Here's the drawing with two shaded views (mm, measured from the low corner). I have some questions. Give positions to 0.01 mm unless a question says otherwise; leave off trailing zeros. Write each loop counter-clockwise with the first axis right and the second up, starting at its lowest first coordinate (ties: lowest second). Pieces come first, ordered by that corner, then holes. Notation, with made-up numbers: (-8.5, 47.5) -> (12.5, 47.5) arc R16 ccw to (12.5, 76.5) -> close; hole circle Ø10 at (86.5, 11.25). An arc over 180 degrees is marked (long way). Put each result on its own line as item: value. Start each with the question number.
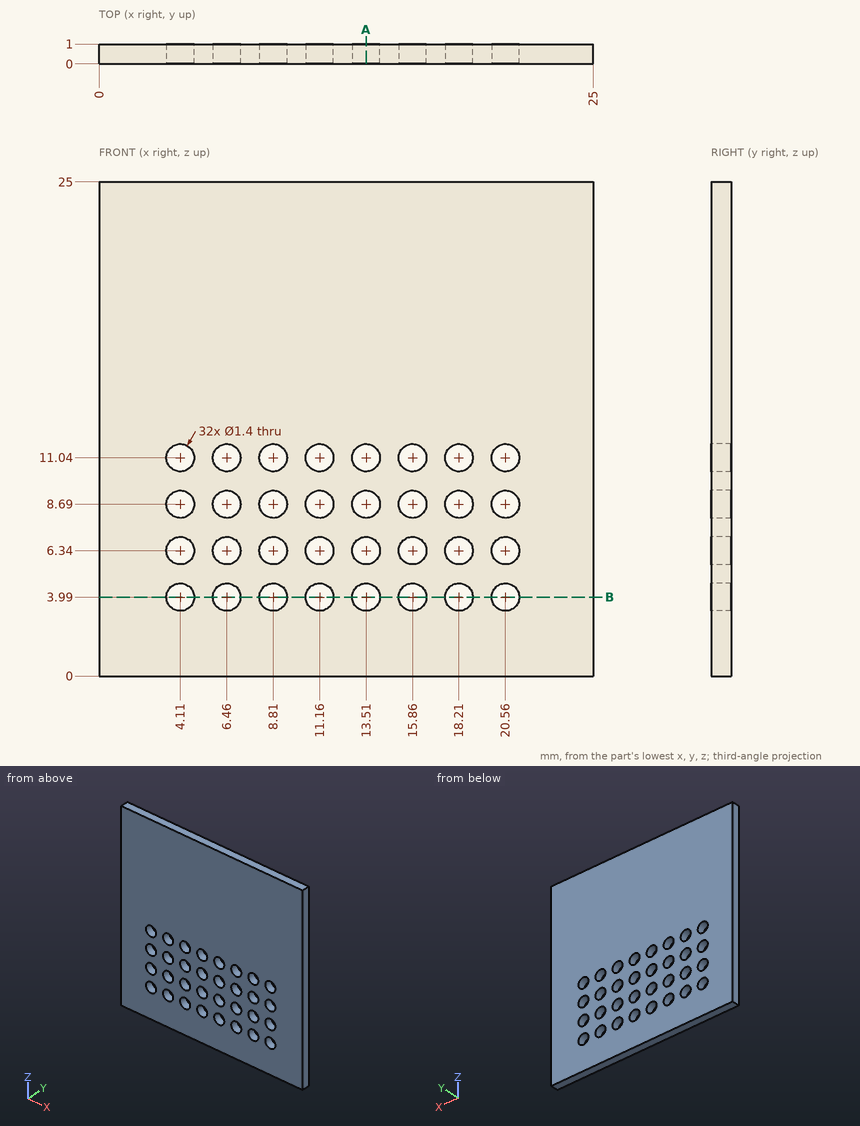
1) I want a section at A-A, the plane x = 13.51. Write out the boundary of the cut face in (y, z), and give its area (3 significant figures).
2) I want a section at B-B, the plane z = 3.99. State how many separate pieces and enclosed holes the cut face has, and give its area (3 significant figures).
3) I need wall thicknesses on probe 1 along Z at (x, y) = (11.16, 0.8); probe 2 along Z at (x, y) = (13, 0.4). Which ranges of each line are inside material? Lowest first, please.
Established:
1. outline: (0, 0) -> (1, 0) -> (1, 3.29) -> (0, 3.29) -> close; (0, 4.69) -> (1, 4.69) -> (1, 5.64) -> (0, 5.64) -> close; (0, 7.04) -> (1, 7.04) -> (1, 7.99) -> (0, 7.99) -> close; (0, 9.39) -> (1, 9.39) -> (1, 10.34) -> (0, 10.34) -> close; (0, 11.74) -> (1, 11.74) -> (1, 25) -> (0, 25) -> close
1. area: 19.4 mm2
2. separate pieces: 9
2. enclosed holes: 0
2. area: 13.8 mm2
3. probe 1: z = 0 to 3.29, 4.69 to 5.64, 7.04 to 7.99, 9.39 to 10.34, 11.74 to 25
3. probe 2: z = 0 to 3.51, 4.47 to 5.86, 6.82 to 8.21, 9.17 to 10.56, 11.52 to 25
